Part model, mm, in its own coordinate system. Coordinates: 2 decimals unless noted, no trailing zeros. Write each loop counter-clockwise with the first axis right and the second up, starting at its lowest first coordinate (ties: lowest second). Pieces come first, ordered by that corner, then holes. Notation, with made-up numbers: (53, -31.75) - (60, -31.75) arc R27 cw to (60, -12.75) - close; hole circle Ø8 at (3.5, 34). An arc over 180 degrees is marked (long way). Use one line per item in the form item = value. Start each with the question number.
Autodesk Fusion 360 part; units mm, degrees
sketch "Sketch1" plane through (0, 0, 0) normal (0, 0, 1) x (1, 0, 0)
  line L0 (125, 46.5) -> (-125, 46.5)
  line L1 (-125, 46.5) -> (-125, -46.5)
  line L2 (-125, -46.5) -> (125, -46.5)
  line L3 (125, -46.5) -> (125, 46.5)
  line L4 (125, 46.5) -> (-125, -46.5) construction
  line L5 (-125, 46.5) -> (125, -46.5) construction
  line L6 (-125, 46.5) -> (-75, 46.5)
  line L7 (-75, 46.5) -> (-75, 43.5)
  line L8 (-75, 43.5) -> (-125, 43.5)
  line L9 (-125, 43.5) -> (-125, 46.5)
  line L10 (25, 43.5) -> (-25, 43.5)
  line L11 (-25, 46.5) -> (25, 46.5)
  line L12 (25, 46.5) -> (25, 43.5)
  line L13 (-25, 43.5) -> (-25, 46.5)
  line L14 (125, 43.5) -> (75, 43.5)
  line L15 (75, 46.5) -> (125, 46.5)
  line L16 (125, 46.5) -> (125, 43.5)
  line L17 (75, 43.5) -> (75, 46.5)
  line L18 (-75, -46.5) -> (-125, -46.5)
  line L19 (-125, -43.5) -> (-75, -43.5)
  line L20 (-75, -43.5) -> (-75, -46.5)
  line L21 (-125, -46.5) -> (-125, -43.5)
  line L22 (25, -46.5) -> (-25, -46.5)
  line L23 (-25, -43.5) -> (25, -43.5)
  line L24 (25, -43.5) -> (25, -46.5)
  line L25 (-25, -46.5) -> (-25, -43.5)
  line L26 (125, -46.5) -> (75, -46.5)
  line L27 (75, -43.5) -> (125, -43.5)
  line L28 (125, -43.5) -> (125, -46.5)
  line L29 (75, -46.5) -> (75, -43.5)
  dimension "d1" = 250
  dimension "d2" = 93
  dimension "d13" = 50
  dimension "d14" = 3
  dimension "d17" = 200
  dimension "d18" = -90
extrude "Extrude3" add sketch "Sketch1" along normal blind 3 contours L0 L1 L2 L3 L7 L8 L10 L12 L13 L14 L17 L19 L20 L23 L24 L25 L27 L29
sketch "Sketch3" plane through (0, 0, 3) normal (0, 0, 1) x (-1, 0, 0)
  line L0 (-75, 46.5) -> (-75, 43.5)
  line L1 (-75, 43.5) -> (-125, 43.5)
  line L2 (-125, 43.5) -> (-125, -43.5)
  line L3 (-125, -43.5) -> (-75, -43.5)
  line L4 (-75, -43.5) -> (-75, -46.5)
  line L5 (-75, -46.5) -> (-25, -46.5)
  line L6 (-25, -46.5) -> (-25, -43.5)
  line L7 (-25, -43.5) -> (25, -43.5)
  line L8 (25, -43.5) -> (25, -46.5)
  line L9 (25, -46.5) -> (75, -46.5)
  line L10 (75, -46.5) -> (75, -43.5)
  line L11 (75, -43.5) -> (125, -43.5)
  line L12 (125, -43.5) -> (125, 43.5)
  line L13 (125, 43.5) -> (75, 43.5)
  line L14 (75, 43.5) -> (75, 46.5)
  line L15 (75, 46.5) -> (25, 46.5)
  line L16 (25, 46.5) -> (25, 43.5)
  line L17 (25, 43.5) -> (-25, 43.5)
  line L18 (-25, 43.5) -> (-25, 46.5)
  line L19 (-25, 46.5) -> (-75, 46.5)
  line L20 (-121.1564, -43.5) -> (-121.1564, -15.5) construction
  line L21 (-121.1564, 43.5) -> (-121.1564, 15.5) construction
  line L22 (-125, -15.5) -> (-122, -15.5)
  line L23 (-122, -15.5) -> (-122, 15.5)
  line L24 (-122, 15.5) -> (-125, 15.5)
  line L25 (-125, 15.5) -> (-125, -15.5)
  dimension "d21" = 28
  dimension "d22" = 28
  dimension "d23" = 3
  dimension "d24" = 31
extrude "Extrude4" cut sketch "Sketch3" against normal blind 6 contours L2 L22 L23 L24 L25
mirror "Mirror1" about plane through (0, 0, 0) normal (1, 0, 0) of "Extrude4"
sketch "Sketch4" plane through (0, 0, 3) normal (0, 0, 1) x (-1, 0, 0)
  line L0 (122, 15.5) -> (125, 15.5)
  line L1 (125, 15.5) -> (125, 43.5)
  line L2 (125, 43.5) -> (75, 43.5)
  line L3 (75, 43.5) -> (75, 46.5)
  line L4 (75, 46.5) -> (25, 46.5)
  line L5 (25, 46.5) -> (25, 43.5)
  line L6 (25, 43.5) -> (-25, 43.5)
  line L7 (-25, 43.5) -> (-25, 46.5)
  line L8 (-25, 46.5) -> (-75, 46.5)
  line L9 (-75, 46.5) -> (-75, 43.5)
  line L10 (-75, 43.5) -> (-125, 43.5)
  line L11 (-125, 43.5) -> (-125, 15.5)
  line L12 (-125, 15.5) -> (-122, 15.5)
  line L13 (-122, 15.5) -> (-122, -15.5)
  line L14 (-122, -15.5) -> (-125, -15.5)
  line L15 (-125, -15.5) -> (-125, -43.5)
  line L16 (-125, -43.5) -> (-75, -43.5)
  line L17 (-75, -43.5) -> (-75, -46.5)
  line L18 (-75, -46.5) -> (-25, -46.5)
  line L19 (-25, -46.5) -> (-25, -43.5)
  line L20 (-25, -43.5) -> (25, -43.5)
  line L21 (25, -43.5) -> (25, -46.5)
  line L22 (25, -46.5) -> (75, -46.5)
  line L23 (75, -46.5) -> (75, -43.5)
  line L24 (75, -43.5) -> (125, -43.5)
  line L25 (125, -43.5) -> (125, -15.5)
  line L26 (125, -15.5) -> (122, -15.5)
  line L27 (122, -15.5) -> (122, 15.5)
Q1. Drill centre lines: probe 1 along X at (y, z) = (7, 1.1); probe 2 along Y at (x, z) = (12.5, 0.35). Where is each one in solid material? Low to high.
Q2. Pin check, flat tips, straight feed: P1, Ø1.5, axis at x = -89.5, z = 1.5, coming from the +Y side; P2, Ø1.5, axis at x = 123, z = 2, coming from the -Y side; P3, Ø0.9, axis at y = -44.5, z = 1.5, coming from the +X side. Stop position of each tip, or through.
Q3. Slice it at C-C (x = -7). List the corners of the cut face in (y, z).
Q4. Slice it at A-A (z = 0.9). List the corners of the cut face in (x, y).
Q5. Slice it at B-B (y = -4.5). List the corners of the cut face in (x, z), plus the area to 3 significant figures.
Solution:
q1.probe_1 = -122 to 122
q1.probe_2 = -43.5 to 43.5
q2.P1 = 43.5
q2.P2 = -43.5
q2.P3 = 75
q3.outline = (-43.5, 0) - (43.5, 0) - (43.5, 3) - (-43.5, 3) - close
q4.outline = (-125, -43.5) - (-75, -43.5) - (-75, -46.5) - (-25, -46.5) - (-25, -43.5) - (25, -43.5) - (25, -46.5) - (75, -46.5) - (75, -43.5) - (125, -43.5) - (125, -15.5) - (122, -15.5) - (122, 15.5) - (125, 15.5) - (125, 43.5) - (75, 43.5) - (75, 46.5) - (25, 46.5) - (25, 43.5) - (-25, 43.5) - (-25, 46.5) - (-75, 46.5) - (-75, 43.5) - (-125, 43.5) - (-125, 15.5) - (-122, 15.5) - (-122, -15.5) - (-125, -15.5) - close
q5.outline = (-122, 0) - (122, 0) - (122, 3) - (-122, 3) - close
q5.area = 732 mm2
